Autodesk Inventor part; units mm, degrees
ref_plane "Work Plane1" through (0, 17, 0) normal (0, -1, 0) x (1, 0, 0)
ref_plane "YZ Plane" through (0, 0, 0) normal (1, 0, 0) x (0, 1, 0)
ref_plane "XZ Plane" through (0, 0, 0) normal (0, 1, 0) x (-1, 0, 0)
sketch "Sketch1" plane through (0, 0, 0) normal (0, 1, 0) x (-1, 0, 0)
  line L0 (-11.45, 6.1) -> (11.45, 6.1)
  line L1 (11.45, 6.1) -> (11.45, -6.1)
  line L2 (11.45, -6.1) -> (-11.45, -6.1)
  line L3 (-11.45, -6.1) -> (-11.45, 6.1)
  line L4 (-11.45, 6.1) -> (11.45, -6.1) construction
  line L5 (11.45, 6.1) -> (-11.45, -6.1) construction
  point P0 (0, 0)
  dimension "d0" = 22.9
  dimension "d1" = 12.2
extrude "Extrusion1" add sketch "Sketch1" along normal blind 28.3
ref_plane "Work Plane1" through (0, 17, 0) normal (0, -1, 0) x (1, 0, 0)
sketch "Sketch2" plane through (0, 17, 0) normal (0, -1, 0) x (1, 0, 0)
  line L0 (-11.45, 6.1) -> (11.45, 6.1)
  line L1 (11.45, 6.1) -> (16.1, 6.1)
  line L2 (16.1, 6.1) -> (16.1, -6.1)
  line L3 (16.1, -6.1) -> (11.45, -6.1)
  line L4 (11.45, -6.1) -> (11.45, 6.1)
  line L5 (-11.45, -6.1) -> (-11.45, 6.1)
  line L6 (-11.45, 6.1) -> (-16.1, 6.1)
  line L7 (-16.1, 6.1) -> (-16.1, 0.65)
  line L8 (-16.1, -6.1) -> (-11.45, -6.1)
  line L9 (-11.45, -6.1) -> (-11.45, 6.1)
  line L10 (11.45, -6.1) -> (-11.45, -6.1)
  arc A0 (-15.05, 0) -> (-14.8758, -0.65) centre (-13.75, 0) ccw construction
  line L11 (-16.1, -0.65) -> (-14.8758, -0.65)
  line L12 (-16.1, 0.65) -> (-14.8758, 0.65)
  line L13 (-16.1, 0) -> (16.1, 0) construction
  line L14 (-16.1, -0.65) -> (-16.1, -6.1)
  line L15 (-16.1, 0.65) -> (-16.1, -0.65) construction
  arc A1 (-14.8758, 0.65) -> (-15.05, 0) centre (-13.75, 0) ccw construction
  arc A2 (-14.8758, -0.65) -> (-14.8758, 0.65) centre (-13.75, 0) ccw
  circle A3 centre (13.75, 0) radius 1.3
  line L16 (14.8758, -0.65) -> (16.1, -0.65)
  line L17 (14.8758, 0.65) -> (16.1, 0.65)
  point P0 (0, 0)
  point P1 (-11.45, 0)
  point P2 (-15.4879, -0.65)
  dimension "d5" = 32.2
  dimension "d6" = 22.9
  dimension "d7" = 4.65
  dimension "d14" = 2.6
  dimension "d15" = 2.3
  dimension "d16" = 1.3
  dimension "d17" = 0.65
  dimension "d18" = 2.6
  dimension "d19" = 2.3
  dimension "d20" = 1.3
  dimension "d21" = 0.65
extrude "Extrusion2" add sketch "Sketch2" against normal blind 2.5 contours L5 L8 L14 L11 A2 L12 L7 L6 | L1 L2 L17 A3 L16 L3 L4
sketch "Sketch3" plane through (0, 28.3, 0) normal (0, 1, 0) x (1, 0, 0)
  circle A0 centre (5.35, 0) radius 2.5
  line L0 (16.1, -6.1) -> (16.1, 6.1)
  line L1 (-11.45, 6.1) -> (-11.45, -6.1) construction
  line L2 (-11.45, 0) -> (16.1, 0)
  circle A1 centre (5.35, 0) radius 6.1 construction
  line L3 (11.45, 6.1) -> (-11.45, 6.1) construction
  line L4 (-11.45, -6.1) -> (11.45, -6.1) construction
  line L5 (11.45, -6.1) -> (11.45, 6.1) construction
  point P0 (0, 0)
  dimension "d10" = 5
extrude "Extrusion3" add sketch "Sketch3" along normal blind 3
sketch "Sketch4" plane through (0, 28.3, 0) normal (0, 1, 0) x (1, 0, 0)
  circle A0 centre (5.35, 0) radius 2.5
  circle A1 centre (5.35, 0) radius 6.1
  circle A2 centre (-0.4, 0) radius 2.65
  line L0 (11.45, 6.1) -> (-11.45, 6.1)
  line L1 (-0.4, 0) -> (5.35, 0)
  line L2 (-0.4, 0) -> (-3.05, 0)
  line L3 (5.35, 0) -> (11.45, 0)
  line L4 (-1.3388, 2.4781) -> (0.0387, 3)
  line L5 (-1.3388, -2.4781) -> (0.0387, -3)
  line L6 (11.45, 6.1) -> (-11.45, 6.1)
  line L7 (11.45, -6.1) -> (11.45, 6.1)
  line L8 (-11.45, -6.1) -> (11.45, -6.1)
  line L9 (-11.45, 6.1) -> (-11.45, -6.1)
  point P0 (0, 0)
  point P1 (5.35, -6.1)
  point P2 (5.35, 6.1)
  dimension "d22" = 14.5
  dimension "d23" = 5.3
  dimension "d24" = 6
  dimension "d25" = 3
extrude "Extrusion4" cut sketch "Sketch4" against normal blind 4.5 contours L7 L8 A1 | A1 L0 L7 | A1 L4 A2 L5 L8 L9 L0
chamfer "Chamfer1" distance 0.5 distance2 4.5 5 edges at (-0.6501, 28.3, 2.7391) (-3.05, 28.3, 0) (-0.6501, 28.3, -2.7391) (10.6183, 28.3, -3.0749) (2.2751, 28.3, 5.2683) measured on face at (0.0574, 28.3, 0)
equation "\"d7\" = -0.5 * d6 + 0.5 * d5"
equation "\"d17\" = 0.5 * d16"
equation "\"d21\" = 0.5 * d20"
properties part number "Servo_small_maketa"
Part model, mm, in its own coordinate system. A direction names the side the tool comes from. Round coordinates to 2 decimals unless told otherwise and drop trailing zeros. Write each loop counter-clockwise with the first axis right and the second up, starting at its lowest first coordinate (ties: lowest second). Pieces come first, ordered by that corner, then holes.
Item 1: Cut at A-A, the plane x = 13.75. Give the cut face in (y, z), plus the area to 3 significant figures.
Results:
outline: (17, -6.1) - (19.5, -6.1) - (19.5, -1.3) - (17, -1.3) - close; (17, 1.3) - (19.5, 1.3) - (19.5, 6.1) - (17, 6.1) - close
area: 24.0 mm2
Item 2: Cut at D-D, the plane y = 15.5. Give the cut face in (x, z).
Results:
outline: (-11.45, -6.1) - (11.45, -6.1) - (11.45, 6.1) - (-11.45, 6.1) - close
Item 3: Drop flat-ended pins along their axis: pin 1 Ø1.3 at (y, z) = (22.5, -1.5) entering from +X; pin 2 Ø4.5 at (y, z) = (22, 1) entering from -X; pin 3 Ø2.5 at (x, z) = (14, 1.5) entering from -Y; pin 4 Ø2.5 at (x, z) = (13.75, 0) entering from +Y. Give the stop position or say it passes through.
Results:
pin 1: stops at x = 11.45
pin 2: stops at x = -11.45
pin 3: stops at y = 17
pin 4: passes through
Item 4: Which spindle directions (+Z, -Z, +X, -X, +Y, -Y) get a long thin tool onto all of the face, cutting with end or side? Do faces 5 (the flat face through (15.5, 18.2, -0.65)), 6 (the flat face through (-15.5, 18.2, 0.65)), 7 (the cylindrical face through (2.852, 29.779, 0.11)). Say none if no direction does.
Results:
face 5: +X, +Y, -Y
face 6: -X, +Y, -Y
face 7: +Y
Item 5: Cut at C-C, the plane x = -11. Give the cut face in (y, z), plus the area to 3 significant figures.
Results:
outline: (0, -6.1) - (23.8, -6.1) - (23.8, 6.1) - (0, 6.1) - close
area: 290 mm2
Item 6: Probe L1, parallel to Z at x = -13.75, y = 19.05; L2, parallel to X at y = 6.5, z = -4; L3, parallel to Y at x = 8.5, z = 3. List the from-to ranges inside material, lowest first.
Results:
L1: z = -6.1 to -1.3, 1.3 to 6.1
L2: x = -11.45 to 11.45
L3: y = 0 to 28.3
Item 7: Two-plate mould, pull along X, no slides. Class faces 1 (the flat face through (11.45, 8, 0)), 2 (the cylindrical face through (12.45, 18.23, 0.05)), 3 (the cylindrical face through (-12.45, 18.23, -0.05)), 4 (the flat face through (10, 23.8, 5)): +X half, -X half, draft (parallel to the pull), parting line (faces both ways), or undercut.
Results:
face 1: +X half
face 2: undercut
face 3: undercut
face 4: draft
Item 8: Cut at B-B, the plane y = 29. Give the cut face in (x, z), plus the area to 3 significant figures.
Results:
outline: circle Ø5 at (5.35, 0)
area: 19.6 mm2
